CAD build for the part. Positions are in the model's coordinates, mm. A direction names the side the tool comes from. Give positions to 0.01 mm unless a question says otherwise; leave off trailing zeros. Order: outer loops, then holes, each group sorted by start corner. A loop starts at its lowest first (then second) coordinate and runs counter-clockwise, first axis right, second up. Notation, with made-up numbers: M 56.25,70 L 95.25,70 A16 cw 95.25,89 Z; hole C -39.75,13 d8. An arc over 180 degrees is marked long. Put each result on its own line as item: value. Start each with the question number.
1) Tool access for faces 1 (the face through (-17, 1, 48)), 2 (the face through (0.13, 6.62, 20.27)): list every direction of +Z, -Z, +X, -X, +Y, -Y with a clear straight run to the whole face (end or side of a thin tool).
2) Drill centre lines: line 1 (X direction, y = 3.5, z = 8.5); line 2 (Z direction, x = 8.5, y = 5.25); line 3 (Z direction, x = 28.5, y = 8). Where is each one in solid material? Low to high. Write a range as [from, to].
3) Pin check, flat tips, straight feed: pin 1 (10 mm diameter, centred on x = -33.5, y = 3.5, fed in from -Z); pin 2 (7.5 mm diameter, centred on x = 20.15, z = 11.63, fed in from +Y); pin 3 (3 mm diameter, centred on x = 34.5, y = 3.5, fed in from +Z); pin 4 (14.5 mm diameter, centred on x = -22, z = 30, fed in from +Y). Stop position of each tip, or through.
4) Two-plate mould, pull along Z, no slides. Class faces 3 (the face through (0, 8, 55.051)), 4 (the face through (-39.98, 7.12, -24.67)), 5 (the face through (0, 8, -55.051)): released by +Z, released by -Z, zero draft, split by the parting line, or undercut.
5) Cut at C-C (x = 11). Write the cut outline in (y, z), and give its area (3 significant figures).
6) Cut at A-A (z = -32). Write the cut outline in (x, y).
7) Cut at B-B (y = 10). Give the number of separate pieces and of enclosed holes in the cut face, and give its area (3 significant figures).
```python
from build123d import *

# Parameters (mm, degrees)
SKETCH1_R           = 13
BOSS_EXTRUDE1_DEPTH = 1
SKETCH2_R           = 14.3125
BOSS_EXTRUDE2_DEPTH = 16.05
SKETCH3_R           = 4.05
CUT_EXTRUDE1_DEPTH  = 4
SKETCH5_R           = 1.55
CUT_EXTRUDE3_DEPTH  = 86.802602692
SKETCH5_3_R         = 2.875
CUT_EXTRUDE4_DEPTH  = 3
SKETCH6_R           = 3
CUT_EXTRUDE5_DEPTH  = 86.09810003


with BuildPart() as part:
    # Sketch1 → Boss-Extrude1 (new body)
    with BuildSketch(Plane(origin=(0, 0, 0), x_dir=(1, 0, 0), z_dir=(0, 1, 0))):
        Polygon((63.567215848, 0), (31.783607924, 55.050823773), (-31.783607924, 55.050823773), (-63.567215848, 0), (-31.783607924, -55.050823773), (31.783607924, -55.050823773), align=None)
        with Locations(Location((0, 0, 0), (0, 0, 270))):
            Circle(SKETCH1_R, mode=Mode.SUBTRACT)
        with Locations(Location((-40.3, 0, 0), (0, 0, 270))):
            Circle(SKETCH1_R, mode=Mode.SUBTRACT)
        with Locations(Location((-20.15, 34.900823773, 0), (0, 0, 270))):
            Circle(SKETCH1_R, mode=Mode.SUBTRACT)
        with Locations(Location((20.15, 34.900823773, 0), (0, 0, 270))):
            Circle(SKETCH1_R, mode=Mode.SUBTRACT)
        with Locations(Location((40.3, 0, 0), (0, 0, 270))):
            Circle(SKETCH1_R, mode=Mode.SUBTRACT)
        with Locations(Location((20.15, -34.900823773, 0), (0, 0, 270))):
            Circle(SKETCH1_R, mode=Mode.SUBTRACT)
        with Locations(Location((-20.15, -34.900823773, 0), (0, 0, 270))):
            Circle(SKETCH1_R, mode=Mode.SUBTRACT)
    extrude(amount=BOSS_EXTRUDE1_DEPTH)

    # Sketch2 → Boss-Extrude2 (add)
    with BuildSketch(Plane(origin=(0, 1, 0), x_dir=(1, 0, 0), z_dir=(0, 1, 0))):
        Polygon((-63.567215848, 0), (-31.783607924, 55.050823773), (31.783607924, 55.050823773), (63.567215848, 0), (31.783607924, -55.050823773), (-31.783607924, -55.050823773), align=None)
        with Locations(Location((-40.3, 0, 0), (0, 0, 270))):
            Circle(SKETCH2_R, mode=Mode.SUBTRACT)
        with Locations(Location((-20.15, 34.900823773, 0), (0, 0, 270))):
            Circle(SKETCH2_R, mode=Mode.SUBTRACT)
        with Locations(Location((20.15, 34.900823773, 0), (0, 0, 270))):
            Circle(SKETCH2_R, mode=Mode.SUBTRACT)
        with Locations(Location((40.3, 0, 0), (0, 0, 270))):
            Circle(SKETCH2_R, mode=Mode.SUBTRACT)
        with Locations(Location((20.15, -34.900823773, 0), (0, 0, 270))):
            Circle(SKETCH2_R, mode=Mode.SUBTRACT)
        with Locations(Location((-20.15, -34.900823773, 0), (0, 0, 270))):
            Circle(SKETCH2_R, mode=Mode.SUBTRACT)
        with Locations(Location((0, 0, 0), (0, 0, 270))):
            Circle(SKETCH2_R, mode=Mode.SUBTRACT)
    extrude(amount=BOSS_EXTRUDE2_DEPTH)

    # Sketch3 → Cut-Extrude1 (cut)
    with BuildSketch(Plane(origin=(0, 17.05, 0), x_dir=(1, 0, 0), z_dir=(0, 1, 0))):
        with Locations(Location((-20.15, 11.633607924, 0), (0, 0, 270))):
            Circle(SKETCH3_R)
        with Locations(Location((0, 23.267215848, 0), (0, 0, 270))):
            Circle(SKETCH3_R)
        with Locations(Location((20.15, 11.633607924, 0), (0, 0, 270))):
            Circle(SKETCH3_R)
        with Locations(Location((20.15, -11.633607924, 0), (0, 0, 270))):
            Circle(SKETCH3_R)
        with Locations(Location((0, -23.267215848, 0), (0, 0, 270))):
            Circle(SKETCH3_R)
        with Locations(Location((-20.15, -11.633607924, 0), (0, 0, 270))):
            Circle(SKETCH3_R)
    extrude(amount=-CUT_EXTRUDE1_DEPTH, mode=Mode.SUBTRACT)

    # Sketch5 → Cut-Extrude3 (cut, through all)
    with BuildSketch(Plane(origin=(0, 17.05, 0), x_dir=(1, 0, 0), z_dir=(0, 1, 0))):
        with Locations(Location((-40.046128973, 23.120643343, 0), (0, 0, 270))):
            Circle(SKETCH5_R)
        with Locations(Location((40.046128973, 23.120643343, 0), (0, 0, 270))):
            Circle(SKETCH5_R)
        with Locations(Location((0, -46.241286685, 0), (0, 0, 270))):
            Circle(SKETCH5_R)
    extrude(amount=-CUT_EXTRUDE3_DEPTH, mode=Mode.SUBTRACT)

    # Sketch5_3 → Cut-Extrude4 (cut)
    with BuildSketch(Plane(origin=(0, 17.05, 0), x_dir=(1, 0, 0), z_dir=(0, 1, 0))):
        with Locations(Location((-40.046128973, 23.120643343, 0), (0, 0, 270))):
            Circle(SKETCH5_3_R)
        with Locations(Location((40.046128973, 23.120643343, 0), (0, 0, 270))):
            Circle(SKETCH5_3_R)
        with Locations(Location((0, -46.241286685, 0), (0, 0, 270))):
            Circle(SKETCH5_3_R)
    extrude(amount=-CUT_EXTRUDE4_DEPTH, mode=Mode.SUBTRACT)

    # Sketch6 → Cut-Extrude5 (cut, through all)
    with BuildSketch(Plane(origin=(0, 13.05, 0), x_dir=(1, 0, 0), z_dir=(0, 1, 0))):
        with Locations(Location((-20.15, -11.633607924, 0), (0, 0, 270))):
            Circle(SKETCH6_R)
        with Locations(Location((-20.15, 11.633607924, 0), (0, 0, 270))):
            Circle(SKETCH6_R)
        with Locations(Location((0, 23.267215848, 0), (0, 0, 270))):
            Circle(SKETCH6_R)
        with Locations(Location((20.15, 11.633607924, 0), (0, 0, 270))):
            Circle(SKETCH6_R)
        with Locations(Location((20.15, -11.633607924, 0), (0, 0, 270))):
            Circle(SKETCH6_R)
        with Locations(Location((0, -23.267215848, 0), (0, 0, 270))):
            Circle(SKETCH6_R)
    extrude(amount=-CUT_EXTRUDE5_DEPTH, mode=Mode.SUBTRACT)


solid = part.part
```
Solution:
1. face 1: +Y
1. face 2: +Y, -Y
2. line 1: [-58.66, -51.82], [-28.78, -11.52], [11.52, 28.78], [51.82, 58.66]
2. line 2: [-55.05, -43.21], [-26.59, -11.52], [11.52, 26.59], [43.21, 55.05]
2. line 3: [-55.05, -46.53], [-23.28, -8.1], [8.1, 23.28], [46.53, 55.05]
3. pin 1: z = -55.05
3. pin 2: y = 13.05
3. pin 3: z = 52.94
3. pin 4: through
4. face 3: released by +Z
4. face 4: undercut
4. face 5: released by -Z
5. outline: M 0,-55.05 L 17.05,-55.05 L 17.05,-45.91 L 1,-45.91 L 1,-44.14 L 0,-44.14 Z; M 0,-25.67 L 1,-25.67 L 1,-23.9 L 17.05,-23.9 L 17.05,-9.16 L 1,-9.16 L 1,-6.93 L 0,-6.93 Z; M 0,6.93 L 1,6.93 L 1,9.16 L 17.05,9.16 L 17.05,23.9 L 1,23.9 L 1,25.67 L 0,25.67 Z; M 0,44.14 L 1,44.14 L 1,45.91 L 17.05,45.91 L 17.05,55.05 L 0,55.05 Z
5. area: 826 mm²
6. outline: M -45.09,0 L -32.82,0 L -32.82,1 L -34.17,1 L -34.17,17.05 L -45.09,17.05 Z; M -7.48,0 L 7.48,0 L 7.48,1 L 6.13,1 L 6.13,17.05 L -6.13,17.05 L -6.13,1 L -7.48,1 Z; M 32.82,0 L 45.09,0 L 45.09,17.05 L 34.17,17.05 L 34.17,1 L 32.82,1 Z
7. separate pieces: 1
7. enclosed holes: 16
7. area: 5,800 mm²
